Could you check a few things on this model? Use its own coordinates, in mm. Face numbers are marked on the shaded views. Give positions to 0.01 mm unless a question says otherwise; leave off trailing zeros. Write each loop counter-clockwise with the first axis right and the second up, starting at its lowest first coordinate (ties: lowest second). Pieces come first, ordered by that corner, then holes. Notation, with made-up numbers: (-29.5, 11) - (1.5, 11) arc R33 cw to (1.5, 40) - close; hole circle Ø7 at (-33, -36.75). An arc over 180 degrees is marked (long way). Answer as CSV lines item,"result". Start each with the question number.
Q1. Will this pin go through, and if not, where does the flat tip stop? pin 1 Ø3 at (y, z) = (11.5, -9.5) entering from +X.
Q2. Imagine slicing it at A-A on z = 0. List the corners of the cut face in (x, y) for me.
Q3. If I drill on line 1 along Z through (x, y) = (2, 11.5); line 2 along Z through (x, y) = (1.35, 0); line 3 along Y through (x, z) = (2.35, 0), over which ranges is the centre line in solid material (lowest first)?
Q4. We'd pull the mould along Z, two halves only. Please class the marked faces 1, 2 and 3: pulls with the +Z half, pulls with the -Z half, needs draft (parallel to the pull), parting line crosses it, or undercut.
Q5. Imagine slicing it at B-B on y = 2. List the corners of the cut face in (x, z) for me.
Q6. Imagine slicing it at C-C on x = 1.4. List the corners of the cut face in (y, z) for me, and give its area (3 significant figures).
Q7. Imagine slicing it at D-D on y = 12. List the corners of the cut face in (x, z) for me, and give its area (3 significant figures).
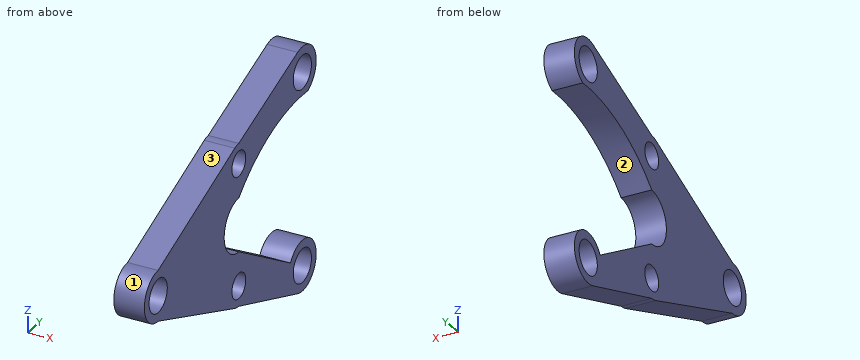
Autodesk Inventor part; units mm, degrees
ref_plane "YZ Plane" through (0, 0, 0) normal (1, 0, 0) x (0, 1, 0)
ref_plane "XZ Plane" through (0, 0, 0) normal (0, 1, 0) x (-1, 0, 0)
ref_plane "XY Plane" through (0, 0, 0) normal (0, 0, 1) x (1, 0, 0)
sketch "スケッチ1" plane through (0, 0, 0) normal (1, 0, 0) x (0, 1, 0)
  line L0 (0, 0) -> (0, 6)
  line L1 (0, 6) -> (0, -6)
  line L2 (0, 0) -> (11.5, 0)
  line L3 (11.5, 0) -> (11.5, 9.5)
  line L4 (11.5, 9.5) -> (11.5, -9.5)
  circle A0 centre (0, 6) radius 1.25
  circle A1 centre (0, -6) radius 1.25
  circle A2 centre (11.5, 9.5) radius 1.65
  circle A3 centre (11.5, -9.5) radius 1.65
  circle A4 centre (11.5, 9.5) radius 2.5
  circle A5 centre (11.5, -9.5) radius 2.5
  circle A6 centre (0, 0) radius 2.65
  line L5 (0, 0) -> (-14.6, 0)
  circle A7 centre (-14.6, 0) radius 1.65
  circle A8 centre (-14.6, 0) radius 2.5
  circle A9 centre (0, 6) radius 2
  circle A10 centre (0, -6) radius 2
  line L6 (0, 8) -> (10.6499, 11.851)
  line L7 (0, -8) -> (10.6499, -11.851)
  line L8 (-14.6, 0) -> (-14.6, -2.5)
  line L9 (-14.6, 0) -> (-12.1, 0) construction
  line L10 (-14.6, -2.5) -> (-14.6, 2.5)
  line L11 (-14.6, -2.5) -> (-0.7212, -7.8655)
  line L12 (-14.6, 2.5) -> (-0.7212, 7.8655)
  circle A11 centre (11.5, -9.5) radius 14.9164
  line L13 (11.5, -9.5) -> (0, 0)
  line L14 (11.5, -9.5) -> (0, -2.65)
  line L15 (14, 9.5) -> (14, 6.6979)
  circle A12 centre (11.5, -9.5) radius 16.7294
  point P0 (9.3522, -8.2206)
  point P1 (0, 2.65)
  point P2 (12.4812, 7.2006)
  dimension "d9" = 5
  dimension "d10" = 5.3
  dimension "d0" = 6
  dimension "d1" = 12
  dimension "d2" = 11.5
  dimension "d3" = 9.5
  dimension "d4" = 19
  dimension "d5" = 2.5
  dimension "d6" = 3.3
  dimension "d7" = 3.3
  dimension "d8" = 5
  dimension "d11" = 14.6
  dimension "d12" = 3.3
  dimension "d13" = 5
  dimension "d14" = 4
  dimension "d15" = 4
  dimension "d16" = 90
extrude "押し出し2" add sketch "スケッチ1" along normal blind 3 contours A6 L5 A8 L12 A9 L0 | L0 A9 L6 A4 A12 | L14 A5 L7 A10 L1 | L1 A10 L11 A11 A6 | A11 L11 A12 A6 | A9 | A6 A12 L11 A8 L5 | A4 A12 | A10 | L14 A3 L4 A5 | A5 L13 A3 L14 | A5 L4 A3 L13 | A8 L8 A7 L5 | L5 A7 L10 A8 | L10 A7 L8 A8
properties part number "ikafly2b"
Conclusion:
1,pin 1,"through"
2,outline,"(0, -17.1) - (3, -17.1) - (3, -16.25) - (0, -16.25) - close; (0, -12.95) - (3, -12.95) - (3, -2.65) - (0, -2.65) - close"
3,line 1,"-12 to -11.15, -7.85 to -7, 7.23 to 7.85, 11.15 to 12"
3,line 2,"-8 to -7.25, -4.75 to -2.65, 2.65 to 4.75, 7.25 to 8"
3,line 3,"-17.1 to -16.25, -12.95 to -2.65"
4,face 1,"parting line crosses it"
4,face 2,"undercut"
4,face 3,"pulls with the +Z half"
5,outline,"(0, -8.72) - (3, -8.72) - (3, -3.84) - (0, -3.84) - close; (0, 4.27) - (3, 4.27) - (3, 8.72) - (0, 8.72) - close"
6,outline,"(-14.6, -2.5) - (-0.72, -7.87) arc R2 ccw to (0, -8) - (10.65, -11.85) arc R2.5 ccw (long way) to (9.35, -8.22) - (0, -2.65) arc R2.65 cw to (0, 2.65) arc R16.73 cw to (12.48, 7.2) arc R2.5 ccw to (10.65, 11.85) - (0, 8) arc R2 ccw to (-0.72, 7.87) - (-14.6, 2.5) arc R2.5 ccw to start; hole circle Ø3.3 at (-14.6, 0); hole circle Ø2.5 at (0, -6); hole circle Ø2.5 at (0, 6); hole circle Ø3.3 at (11.5, -9.5); hole circle Ø3.3 at (11.5, 9.5)"
6,area,"237 mm^2"
7,outline,"(0, -11.95) - (3, -11.95) - (3, -11.07) - (0, -11.07) - close; (0, -7.93) - (3, -7.93) - (3, -7.05) - (0, -7.05) - close; (0, 7.22) - (3, 7.22) - (3, 7.93) - (0, 7.93) - close; (0, 11.07) - (3, 11.07) - (3, 11.95) - (0, 11.95) - close"
7,area,"10.0 mm^2"
